Can you work these out from the model? Positions are in its coordinate system, mm. A direction names the side the tool comes from. Give positions to 0.01 mm unless a question says otherwise; leave off trailing zeros. Loops run counter-clockwise (first coordinate to the right, second up) from the corner with the lowest first, then second, coordinate; pieces in that order, holes last. Notation, with made-up numbers: (36, -35.5) - (54, -35.5) arc R12 ccw to (54, -16.5) - close; hole circle Ø1 at (13, 41). An arc over 180 degrees is marked (long way). Answer as a JSON object with one key per item and string values. Group by question number.
Item 1: Suppose I cut it at C-C on y = -1.5. Write out the boundary of the cut face in (x, z).
Item 2: Will these pins go through, and if not, where does the flat tip stop? pin 1 (4.5 mm diameter, centred on y = 3, z = -8.5, fed in from -X); pin 2 (3 mm diameter, centred on x = 3, z = 7.5, fed in from +Y); pin 3 (1.8 mm diameter, centred on x = 3.5, y = -1, fed in from -Z).
Item 3: Suppose I cut it at A-A on z = 7.5. Write out the boundary of the cut face in (x, y).
Item 4: Suppose I cut it at D-D on y = 8.5. Write out the boundary of the cut face in (x, z).
Item 5: Suppose I cut it at B-B on x = 3. Count the separate pieces of the cut face and the enclosed holes in it, and give its area (3 significant figures).
Item 6: Please list where these lines run through material, in increasing order: L1, parallel to Y at x = 2.35, z = 7.75; L2, parallel to Z at x = 3, y = 6.75; L3, parallel to Z at x = 5.1, y = 6.
Item 7: Which directions (+Z, -Z, +X, -X, +Y, -Y) give clear straight access to the entire face, cutting with the end or side of a thin tool? Please do faces 1 (the flat face through (0, 0, 0)), 2 (the flat face through (3, -7, 6.5)), 3 (the flat face through (3, 7, 6.5)), 4 (the flat face through (3, 6.5, 6.5)).
Item 8: Thinking about a two-plate mould opening in Z: for faces 5 (the flat face through (3, -6.5, 6.5)), 6 (the flat face through (3, 0, 5)), 7 (the cylindrical face through (3.15, 6.747, 7.977)), which applies, pulls with the +Z half, pulls with the -Z half, needs draft (parallel to the pull), parting line crosses it, or undercut?
from build123d import *

# Parameters (mm, degrees)
SKETCH1_W               = 10
SKETCH1_H               = 20
BOSS_EXTRUDE1_DEPTH     = 6
SKETCH2_W               = 3
SKETCH2_H               = 0.5
BOSS_EXTRUDE2_DEPTH     = 4
FILLET1_R               = 0.5
CUT_EXTRUDE1_DEPTH      = 21.14944168
CUT_EXTRUDE1_DEPTH_BACK = 21.14944168
SKETCH3_R               = 0.5
BOSS_EXTRUDE3_DEPTH     = 2
FILLET2_R               = 0.5
FILLET3_R               = 0.125


with BuildPart() as part:
    # Sketch1 → Boss-Extrude1 (new body)
    with BuildSketch(Plane(origin=(0, 0, 0), x_dir=(0, 0, -1), z_dir=(1, 0, 0))):
        Rectangle(SKETCH1_W, SKETCH1_H)
    extrude(amount=BOSS_EXTRUDE1_DEPTH)

    # Sketch2 → Boss-Extrude2 (add)
    with BuildSketch(Plane.XY.offset(5)):
        with Locations((3, 6.75)):
            Rectangle(SKETCH2_W, SKETCH2_H)
        with Locations((3, -6.75)):
            Rectangle(SKETCH2_W, SKETCH2_H)
    extrude(amount=BOSS_EXTRUDE2_DEPTH)

    # Fillet1
    fillet1_edges = [part.edges().sort_by_distance(p)[0] for p in [
        (1.5, 6.75, 5),
        (4.5, 6.75, 5),
        (1.5, 6.75, 9),
        (4.5, 6.75, 9),
        (1.5, -6.75, 5),
        (4.5, -6.75, 5),
        (1.5, -6.75, 9),
        (4.5, -6.75, 9),
    ]]
    fillet(fillet1_edges, radius=FILLET1_R)

    # Sketch3 → Cut-Extrude1 (cut, two sides: drawn at the far end of the back side and taken through both)
    with BuildSketch(Plane(origin=(0, 7, 0), x_dir=(1, 0, 0), z_dir=(0, 1, 0)).offset(-CUT_EXTRUDE1_DEPTH_BACK)):
        with Locations(Location((3, -7.5, 0), (0, 0, 270))):
            Circle(SKETCH3_R)
    extrude(amount=CUT_EXTRUDE1_DEPTH + CUT_EXTRUDE1_DEPTH_BACK, mode=Mode.SUBTRACT)

    # Sketch4 → Boss-Extrude3 (add, symmetric)
    with BuildSketch(Plane(origin=(3, 0, 0), x_dir=(0, 0, -1), z_dir=(1, 0, 0))):
        Polygon((5, 7), (5.5, 7), (10.59558328, -7), (10.478121702, -7.042752518), (5.412474058, 6.875), (5, 6.875), (4.5, 6.875), (4.5, 7), align=None)
    extrude(amount=BOSS_EXTRUDE3_DEPTH, both=True)

    # Fillet2
    fillet2_edges = [part.edges().sort_by_distance(p)[0] for p in [
        (3, 7, -5.5),
        (3, 6.875, -5.412474058),
    ]]
    fillet(fillet2_edges, radius=FILLET2_R)

    # Fillet3
    # the kernel refuses this fillet: 0.125 mm, written as the material it adds along each edge
    with BuildSketch(Plane(origin=(1, 6.875, -5), x_dir=(-1, 0, 0), z_dir=(0, 1, 0)), Plane(origin=(5, 6.875, -5), x_dir=(0, 0, -1), z_dir=(0, 1, 0))) as fillet3_piece_1:
        with BuildLine():
            CenterArc((FILLET3_R, -FILLET3_R), FILLET3_R, 90, 90)
            Line((0, -FILLET3_R), (-FILLET3_R * 0.02, -FILLET3_R))
            Line((-FILLET3_R * 0.02, -FILLET3_R), (-FILLET3_R * 0.02, FILLET3_R * 0.02))
            Line((-FILLET3_R * 0.02, FILLET3_R * 0.02), (FILLET3_R, FILLET3_R * 0.02))
            Line((FILLET3_R, FILLET3_R * 0.02), (FILLET3_R, 0))
        make_face()
    extrude(amount=0.125)
    with BuildSketch(Plane(origin=(1, 6.875, -5), x_dir=(0, -1, 0), z_dir=(1, 0, 0))) as fillet3_piece_2:
        with BuildLine():
            CenterArc((0.130266962, 0.125), FILLET3_R, 170.385831611, 99.614168389)
            Line((0.007022616, 0.14587657), (-0.005301818, 0.147964228))
            ThreePointArc((-0.005301818, 0.147964228), (-0.0125, 0.062370289), (-0.0125, 0))
            Line((-0.0125, 0), (0, -0.0125))
            Line((0, -0.0125), (0.130266962, -0.0125))
            Line((0.130266962, -0.0125), (0.130266962, 0))
        make_face()
    extrude(amount=4)
    with BuildSketch(Plane(origin=(5, 7, -5), x_dir=(0, 0, -1), z_dir=(-1, 0, 0))) as fillet3_piece_3:
        with BuildLine():
            CenterArc((FILLET3_R, -FILLET3_R), FILLET3_R, 90, 90)
            Line((0, -FILLET3_R), (-FILLET3_R * 0.02, -FILLET3_R))
            Line((-FILLET3_R * 0.02, -FILLET3_R), (-FILLET3_R * 0.02, FILLET3_R * 0.02))
            Line((-FILLET3_R * 0.02, FILLET3_R * 0.02), (FILLET3_R, FILLET3_R * 0.02))
            Line((FILLET3_R, FILLET3_R * 0.02), (FILLET3_R, 0))
        make_face()
    extrude(amount=4)
    with BuildSketch(Plane(origin=(0.634886225, 6.875, -5), x_dir=(0, -1, 0), z_dir=(1, 0, 0))) as fillet3_piece_4a_section:
        with BuildLine():
            CenterArc((0.130266962, 0.125), FILLET3_R, 170.385831611, 99.614168389)
            Line((0.007022616, 0.14587657), (-0.005301818, 0.147964228))
            ThreePointArc((-0.005301818, 0.147964228), (-0.0125, 0.062370289), (-0.0125, 0))
            Line((-0.0125, 0), (0, -0.0125))
            Line((0, -0.0125), (0.130266962, -0.0125))
            Line((0.130266962, -0.0125), (0.130266962, 0))
        make_face()
    fillet3_piece_4a = extrude(amount=4.365113775, mode=Mode.PRIVATE)
    fillet3_piece_4a = split(fillet3_piece_4a, bisect_by=Plane(origin=(1, 6.846895643, -5.033240906), z_dir=(-1, 0, 0)), keep=Keep.TOP, mode=Mode.PRIVATE)
    with BuildSketch(Plane(origin=(1, 6.5625, -5), x_dir=(-1, 0, 0), z_dir=(0, 1, 0))) as fillet3_piece_4b_section:
        with BuildLine():
            CenterArc((FILLET3_R, -FILLET3_R), FILLET3_R, 90, 90)
            Line((0, -FILLET3_R), (-FILLET3_R * 0.02, -FILLET3_R))
            Line((-FILLET3_R * 0.02, -FILLET3_R), (-FILLET3_R * 0.02, FILLET3_R * 0.02))
            Line((-FILLET3_R * 0.02, FILLET3_R * 0.02), (FILLET3_R, FILLET3_R * 0.02))
            Line((FILLET3_R, FILLET3_R * 0.02), (FILLET3_R, 0))
        make_face()
    fillet3_piece_4b = extrude(amount=0.4375, mode=Mode.PRIVATE)
    fillet3_piece_4b = split(fillet3_piece_4b, bisect_by=Plane(origin=(0.971700611, 6.875, -5.028299389), z_dir=(0, -1, 0)), keep=Keep.TOP, mode=Mode.PRIVATE)
    fillet3_piece_4 = fillet3_piece_4a & fillet3_piece_4b
    add(fillet3_piece_4)
    with BuildSketch(Plane(origin=(5, 7, -5), x_dir=(0, 0, -1), z_dir=(-1, 0, 0))) as fillet3_piece_5a_section:
        with BuildLine():
            CenterArc((FILLET3_R, -FILLET3_R), FILLET3_R, 90, 90)
            Line((0, -FILLET3_R), (-FILLET3_R * 0.02, -FILLET3_R))
            Line((-FILLET3_R * 0.02, -FILLET3_R), (-FILLET3_R * 0.02, FILLET3_R * 0.02))
            Line((-FILLET3_R * 0.02, FILLET3_R * 0.02), (FILLET3_R, FILLET3_R * 0.02))
            Line((FILLET3_R, FILLET3_R * 0.02), (FILLET3_R, 0))
        make_face()
    fillet3_piece_5a = extrude(amount=4.3125, mode=Mode.PRIVATE)
    fillet3_piece_5a = split(fillet3_piece_5a, bisect_by=Plane(origin=(1, 7.028299389, -5.028299389), z_dir=(-1, 0, 0)), keep=Keep.TOP, mode=Mode.PRIVATE)
    with BuildSketch(Plane(origin=(1, 6.875, -5), x_dir=(-1, 0, 0), z_dir=(0, 1, 0))) as fillet3_piece_5b_section:
        with BuildLine():
            CenterArc((FILLET3_R, -FILLET3_R), FILLET3_R, 90, 90)
            Line((0, -FILLET3_R), (-FILLET3_R * 0.02, -FILLET3_R))
            Line((-FILLET3_R * 0.02, -FILLET3_R), (-FILLET3_R * 0.02, FILLET3_R * 0.02))
            Line((-FILLET3_R * 0.02, FILLET3_R * 0.02), (FILLET3_R, FILLET3_R * 0.02))
            Line((FILLET3_R, FILLET3_R * 0.02), (FILLET3_R, 0))
        make_face()
    fillet3_piece_5b = extrude(amount=0.4375, mode=Mode.PRIVATE)
    fillet3_piece_5b = split(fillet3_piece_5b, bisect_by=Plane(origin=(0.971700611, 7, -5.028299389), z_dir=(0, 1, 0)), keep=Keep.TOP, mode=Mode.PRIVATE)
    fillet3_piece_5 = fillet3_piece_5a & fillet3_piece_5b
    add(fillet3_piece_5)
    with BuildSketch(Plane(origin=(5, 6.5625, -5), x_dir=(0, 0, -1), z_dir=(0, 1, 0))) as fillet3_piece_6a_section:
        with BuildLine():
            CenterArc((FILLET3_R, -FILLET3_R), FILLET3_R, 90, 90)
            Line((0, -FILLET3_R), (-FILLET3_R * 0.02, -FILLET3_R))
            Line((-FILLET3_R * 0.02, -FILLET3_R), (-FILLET3_R * 0.02, FILLET3_R * 0.02))
            Line((-FILLET3_R * 0.02, FILLET3_R * 0.02), (FILLET3_R, FILLET3_R * 0.02))
            Line((FILLET3_R, FILLET3_R * 0.02), (FILLET3_R, 0))
        make_face()
    fillet3_piece_6a = extrude(amount=0.4375, mode=Mode.PRIVATE)
    fillet3_piece_6a = split(fillet3_piece_6a, bisect_by=Plane(origin=(5.028299389, 6.875, -5.028299389), z_dir=(0, -1, 0)), keep=Keep.TOP, mode=Mode.PRIVATE)
    with BuildSketch(Plane(origin=(1, 6.875, -5), x_dir=(0, -1, 0), z_dir=(1, 0, 0))) as fillet3_piece_6b_section:
        with BuildLine():
            CenterArc((0.130266962, 0.125), FILLET3_R, 170.385831611, 99.614168389)
            Line((0.007022616, 0.14587657), (-0.005301818, 0.147964228))
            ThreePointArc((-0.005301818, 0.147964228), (-0.0125, 0.062370289), (-0.0125, 0))
            Line((-0.0125, 0), (0, -0.0125))
            Line((0, -0.0125), (0.130266962, -0.0125))
            Line((0.130266962, -0.0125), (0.130266962, 0))
        make_face()
    fillet3_piece_6b = extrude(amount=4.365113775, mode=Mode.PRIVATE)
    fillet3_piece_6b = split(fillet3_piece_6b, bisect_by=Plane(origin=(5, 6.846895643, -5.033240906), z_dir=(1, 0, 0)), keep=Keep.TOP, mode=Mode.PRIVATE)
    fillet3_piece_6 = fillet3_piece_6a & fillet3_piece_6b
    add(fillet3_piece_6)
    with BuildSketch(Plane(origin=(5, 6.875, -5), x_dir=(0, 0, -1), z_dir=(0, 1, 0))) as fillet3_piece_7a_section:
        with BuildLine():
            CenterArc((FILLET3_R, -FILLET3_R), FILLET3_R, 90, 90)
            Line((0, -FILLET3_R), (-FILLET3_R * 0.02, -FILLET3_R))
            Line((-FILLET3_R * 0.02, -FILLET3_R), (-FILLET3_R * 0.02, FILLET3_R * 0.02))
            Line((-FILLET3_R * 0.02, FILLET3_R * 0.02), (FILLET3_R, FILLET3_R * 0.02))
            Line((FILLET3_R, FILLET3_R * 0.02), (FILLET3_R, 0))
        make_face()
    fillet3_piece_7a = extrude(amount=0.4375, mode=Mode.PRIVATE)
    fillet3_piece_7a = split(fillet3_piece_7a, bisect_by=Plane(origin=(5.028299389, 7, -5.028299389), z_dir=(0, 1, 0)), keep=Keep.TOP, mode=Mode.PRIVATE)
    with BuildSketch(Plane(origin=(5.3125, 7, -5), x_dir=(0, 0, -1), z_dir=(-1, 0, 0))) as fillet3_piece_7b_section:
        with BuildLine():
            CenterArc((FILLET3_R, -FILLET3_R), FILLET3_R, 90, 90)
            Line((0, -FILLET3_R), (-FILLET3_R * 0.02, -FILLET3_R))
            Line((-FILLET3_R * 0.02, -FILLET3_R), (-FILLET3_R * 0.02, FILLET3_R * 0.02))
            Line((-FILLET3_R * 0.02, FILLET3_R * 0.02), (FILLET3_R, FILLET3_R * 0.02))
            Line((FILLET3_R, FILLET3_R * 0.02), (FILLET3_R, 0))
        make_face()
    fillet3_piece_7b = extrude(amount=4.3125, mode=Mode.PRIVATE)
    fillet3_piece_7b = split(fillet3_piece_7b, bisect_by=Plane(origin=(5, 7.028299389, -5.028299389), z_dir=(1, 0, 0)), keep=Keep.TOP, mode=Mode.PRIVATE)
    fillet3_piece_7 = fillet3_piece_7a & fillet3_piece_7b
    add(fillet3_piece_7)


solid = part.part
Worked out:
{
 "1": {"outline": "(0, -5) - (6, -5) - (6, 5) - (0, 5) - close; (1, -8.59) - (5, -8.59) - (5, -8.46) - (1, -8.46) - close"},
 "2": {"pin 1": "stops at x = 1", "pin 2": "stops at y = 7", "pin 3": "stops at z = -8.74"},
 "3": {"outline": "(1.5, -7) - (2.5, -7) - (2.5, -6.5) - (1.5, -6.5) - close; (1.5, 6.5) - (2.5, 6.5) - (2.5, 7) - (1.5, 7) - close; (3.5, -7) - (4.5, -7) - (4.5, -6.5) - (3.5, -6.5) - close; (3.5, 6.5) - (4.5, 6.5) - (4.5, 7) - (3.5, 7) - close"},
 "4": {"outline": "(0, -5) - (6, -5) - (6, 5) - (0, 5) - close"},
 "5": {"separate pieces": "3", "enclosed holes": "0", "area": "205 mm2"},
 "6": {"L1": "y = -7 to -6.5, 6.5 to 7", "L2": "z = -5.58 to -5.39, -5 to 7, 8 to 9", "L3": "z = -5 to 5"},
 "7": {"face 1": "+Z, -Z, -X, +Y, -Y", "face 2": "+Z, +X, -X, -Y", "face 3": "+Z, +X, -X, +Y", "face 4": "+Z, +X, -X"},
 "8": {"face 5": "needs draft", "face 6": "pulls with the +Z half", "face 7": "undercut"}
}
